Read the model definition and answer for the solid it produces. Units are mm, in the model's axes. A direction names the side the tool comes from. Round coordinates to 2 decimals unless told otherwise and drop trailing zeros. Order: outer loops, then holes, each group sorted by start corner. A loop starts at its lowest first (then second) coordinate and runs counter-clockwise, first axis right, second up. Notation, with made-up numbers: (29.25, 81) -> (34.25, 81) arc R20 cw to (34.25, 94) -> close; hole circle Ø11 at (29, 19). An arc over 180 degrees is marked (long way). Answer as a JSON object with one key per item and string values. Group by question number.
Item 1: For faces 1 (the cylindrical face through (-0.053, -1.743, -10.5)), 2 (the flat face through (0, -6, -7.281)), 3 (the flat face through (0, -1, 4.4)), determine the directions among +Z, -Z, +X, -X, +Y, -Y from which every point of the face is accessible in a straight line to the end or side of a thin tool.
Item 2: Section B-B, the plane z = -6.9 is taken. Write down the section's boundary in (x, y).
Item 3: Section D-D, the plane y = 2 is taken. Write down the section's boundary in (x, z).
Item 4: The mould has two halves that part along Y. Classify faces 4 (the cylindrical face through (-0.053, -3.111, 4.304)), 5 (the cylindrical face through (0.575, -4.014, -8.286)), 6 (the flat face through (0, -2, -3.2)), 7 (the flat face through (0, -7.851, -6)): pulls with the +Y half, pulls with the -Y half, needs draft (parallel to the pull), parting line crosses it, or undercut.
Item 5: Consider probe 1 along Z at (x, y) = (2, -2.5); probe 2 along Z at (x, y) = (-0.75, -1); probe 3 along Y at (x, z) = (0.5, -4.75). Determine where each line is inside the solid, lowest interval first. Write a range as from..to.
Item 6: Given P1, Ø1.1, axis at x = -1, z = -8, coming from the +Y side; P2, Ø1.5, axis at x = 0.5, y = -1, coming from the +Z side; P3, Ø1, axis at x = 0.5, y = 2, coming from the +Z side, each flat-ended and moving along its own axis, determine where each tip first touches the part or whether it passes through.
Item 7: Section A-A, the plane y = -1 is taken. Write down the section's boundary in (x, z).
Item 8: Section C-C, the plane x = 2.5 is taken. Write down the section's boundary in (y, z).
from build123d import *

# Parameters (mm, degrees)
BASE_EXTRUDE_DEPTH      = 3.8
CUT_EXTRUDE1_DEPTH      = 15.038454366
CUT_EXTRUDE1_DEPTH_BACK = 15.038454366


with BuildPart() as part:
    # Sketch1 → Base-Extrude (new, symmetric)
    with BuildSketch(Plane.ZY):
        with BuildLine():
            Line((-9.65, -2), (-4.4, -2))
            Line((-4.4, -2), (-4.4, 0))
            ThreePointArc((-4.4, 0), (0, 4.4), (4.4, 0))
            Line((4.4, 0), (4.4, -1.85))
            ThreePointArc((4.4, -1.85), (4.285410197, -3.120820393), (3.2, -2.45))
            Line((3.2, -2.45), (3.2, 0))
            ThreePointArc((3.2, 0), (0, 3.2), (-3.2, 0))
            Line((-3.2, 0), (-3.2, -3.2))
            Line((-3.2, -3.2), (-11, -3.2))
            Line((-11, -3.2), (-11, -2.45))
            ThreePointArc((-11, -2.45), (-10.487170825, -1.738487526), (-9.65, -2))
        make_face()
    extrude(amount=BASE_EXTRUDE_DEPTH, both=True)

    # Sketch4 → Boss-Revolve1 (revolve)
    with BuildSketch(Plane.ZY, mode=Mode.PRIVATE) as boss_revolve1_sk:
        Polygon((-6.9, -3.2), (-6.9, -7.851), (-5.63, -7.851), (-5.15, -4.851), (-5.4, -4.851), (-5.4, -3.2), align=None)
    revolve(boss_revolve1_sk.sketch.rotate(Axis((0, -3.2, -6.9), (0, 1, 0)), 180), axis=Axis((0, -3.2, -6.9), (0, 1, 0)))

    # Sketch5 → Cut-Extrude1 (cut, two sides: drawn at the far end of the back side and taken through both)
    with BuildSketch(Plane.ZY.offset(-CUT_EXTRUDE1_DEPTH_BACK)):
        with BuildLine():
            Line((-7.281, -7.851), (-6.519, -7.851))
            Line((-6.519, -7.851), (-6.519, -3.787))
            ThreePointArc((-6.519, -3.787), (-6.9, -3.406), (-7.281, -3.787))
            Line((-7.281, -3.787), (-7.281, -7.851))
        make_face()
    extrude(amount=CUT_EXTRUDE1_DEPTH + CUT_EXTRUDE1_DEPTH_BACK, mode=Mode.SUBTRACT)


solid = part.part
Values found:
{
 "1": {"face 1": "+X, -X, +Y", "face 2": "+X, -X, -Y", "face 3": "+Z, +X, -X, +Y"},
 "2": {"outline": "(-3.8, -3.2) -> (-1.5, -3.2) -> (-1.5, -3.41) -> (1.5, -3.41) -> (1.5, -3.2) -> (3.8, -3.2) -> (3.8, -2) -> (-3.8, -2) -> close"},
 "3": {"outline": "(-3.8, -3.92) -> (3.8, -3.92) -> (3.8, -2.5) -> (-3.8, -2.5) -> close; (-3.8, 2.5) -> (3.8, 2.5) -> (3.8, 3.92) -> (-3.8, 3.92) -> close"},
 "4": {"face 4": "parting line crosses it", "face 5": "undercut", "face 6": "needs draft", "face 7": "pulls with the -Y half"},
 "5": {"probe 1": "-11..-3.2, 3.2..4.7", "probe 2": "-4.4..-3.2, 3.2..4.4", "probe 3": "-3.2..-2"},
 "6": {"P1": "y = -2", "P2": "z = 4.4", "P3": "z = 4.14"},
 "7": {"outline": "(-3.8, -4.4) -> (3.8, -4.4) -> (3.8, -3.2) -> (-3.8, -3.2) -> close; (-3.8, 3.2) -> (3.8, 3.2) -> (3.8, 4.4) -> (-3.8, 4.4) -> close"},
 "8": {"outline": "(-3.2, -11) -> (-2.45, -11) arc R0.75 ccw to (-2, -9.65) -> (-2, -4.4) -> (0, -4.4) arc R4.4 ccw to (0, 4.4) -> (-1.85, 4.4) arc R0.75 ccw (long way) to (-2.45, 3.2) -> (0, 3.2) arc R3.2 cw to (0, -3.2) -> (-3.2, -3.2) -> close"}
}
